Autodesk Inventor part; units mm, degrees
ref_plane "YZ Plane" through (0, 0, 0) normal (1, 0, 0) x (0, 1, 0)
ref_plane "XZ Plane" through (0, 0, 0) normal (0, 1, 0) x (-1, 0, 0)
ref_plane "XY Plane" through (0, 0, 0) normal (0, 0, 1) x (1, 0, 0)
sketch "Sketch1" plane through (0, 0, 0) normal (0, 0, 1) x (1, 0, 0)
  circle A0 centre (0, 0) radius 3.175
  dimension "d0" = 6.35
extrude "Extrusion1" add sketch "Sketch1" along normal blind 38.1
sketch "Sketch2" plane through (0, 0, 38.1) normal (0, 0, 1) x (1, 0, 0)
  line L0 (5.693, 0) -> (2.8465, -4.9303)
  line L1 (2.8465, -4.9303) -> (-2.8465, -4.9303)
  line L2 (-2.8465, -4.9303) -> (-5.693, 0)
  line L3 (-5.693, 0) -> (-2.8465, 4.9303)
  line L4 (-2.8465, 4.9303) -> (2.8465, 4.9303)
  line L5 (2.8465, 4.9303) -> (5.693, 0)
  point P0 (0, 0)
  point P1 (0, 0)
extrude "Extrusion2" add sketch "Sketch2" against normal blind 3.9688
chamfer "Chamfer1" distance 0.254 angle 45 1 edges at (-3.175, 0, 0)
properties part number "1.5in bolt"
Here's how the part is built. I have some questions about the finished solid (model axes, mm). A direction names the side the tool comes from. Round coordinates to 2 decimals unless told otherwise and drop trailing zeros. Order: outer loops, then holes, each group sorted by start corner. A loop starts at its lowest first (then second) coordinate and runs counter-clockwise, first axis right, second up. Notation, with made-up numbers: M 69.5,32.5 L 95.5,32.5 A26 ccw 95.5,65.5 Z; hole C 76.25,1 d3. An arc over 180 degrees is marked long. One line per question, with ' | ' between items.
1) I want a section at A-A, the plane z = 35. Write out the boundary of the cut face in (x, y).
Working result:
outline: M -5.69,0 L -2.85,-4.93 L 2.85,-4.93 L 5.69,0 L 2.85,4.93 L -2.85,4.93 Z
2) For faces 1 (the face through (-0.69, 3.1, 16.96)), 2 (the face through (4.29, -2.43, 36.14)), which set-ups out of +Z, -Z, +X, -X, +Y, -Y let a thin tool reach every point of the face, with its end or its side?
Working result:
face 1: -Z | face 2: +Z, -Z, +X, -Y
3) I need wall thicknesses on line 1 along X through (y, z) = (0, 17) (3 decimals); line 2 along Z through (x, y) = (2, -2.5); line 3 along X through (y, z) = (1.25, 20). Which ranges of each line are inside material? Lowest first, please.
Working result:
line 1: -3.175 to 3.175 | line 2: 34.13 to 38.1 | line 3: -2.92 to 2.92
4) I want a section at D-D, the plane z = 25.5. Write out the boundary of the cut face in (x, y) (3 decimals).
Working result:
outline: C 0,0 d6.35
5) I want a section at B-B, the plane x = 0. Write out the boundary of the cut face in (y, z) (3 decimals), then the cut area to 3 significant figures.
Working result:
outline: M -4.93,34.131 L -3.175,34.131 L -3.175,0.254 L -2.921,0 L 2.921,0 L 3.175,0.254 L 3.175,34.131 L 4.93,34.131 L 4.93,38.1 L -4.93,38.1 Z | area: 256 mm²
6) I want a section at C-C, the plane y = 4. Write out the boundary of the cut face in (x, z), then the cut area to 3 significant figures.
Working result:
outline: M -3.38,34.13 L 3.38,34.13 L 3.38,38.1 L -3.38,38.1 Z | area: 26.9 mm²
7) For pin 1 Ø1 at (x, z) = (0.5, 21.5) entering from +Y (3 decimals); pin 2 Ø2 at (x, z) = (-4.5, 31) entering from -Y, each with a flat end and sliding along its axis, tell me the tip position at first contact or that it passes through.
Working result:
pin 1: y = 3.175 | pin 2: through
